Here's how the part is built. I have some questions about the finished solid (model axes, mm). Give positions to 0.01 mm unless a question says otherwise; leave off trailing zeros. Loops run counter-clockwise (first coordinate to the right, second up) from the corner with the lowest first, then second, coordinate; pieces in that order, holes last. Notation, with made-up numbers: (24, -40) -> (34, -40) arc R9 cw to (34, -32) -> close; hole circle Ø3 at (47, 32). An arc over 180 degrees is marked (long way). Answer in a Markdown table with one row per item. Add a question column.
Item 1: If I drill on line 1 (Y direction, x = 0, z = 0.3); line 2 (X direction, y = -1, z = 0.3); line 3 (X direction, y = 2, z = 0.9), over which ranges is the centre line in solid material (lowest first)?
Item 2: We'd pull the mould along X, two halves only. Please class faces 1 (the face through (0, -4, 1.05)), 2 (the face through (4.74, -2.79, 0.01)), 3 (the face through (-4.785, -2.712, 0.014)), 4 (the face through (0.45, 3.425, -0.015)): released by +X, released by -X, zero draft, split by the parting line, or undercut.
Item 3: If we section it at B-B (z = -0.05): Write out the boundary of the cut face in (x, y), then the cut area to 3 significant figures.
Item 4: If we section it at A-A (x = 0): Write out the boundary of the cut face in (y, z), then the cut area to 3 significant figures.
```python
from build123d import *

# Parameters (mm, degrees)
BOSS_EXTRUDE1_DEPTH      = 1.05
F_5_16_24_TAPPED_HOLE1_D = 6.9088


with BuildPart() as part:
    # Sketch2 → Boss-Extrude1 (new body, symmetric)
    with BuildSketch(Plane.XY):
        Polygon((-3.175426481, -5.5), (3.175426481, -5.5), (6.350852961, 0), (3.175426481, 5.5), (-3.175426481, 5.5), (-6.350852961, 0), align=None)
    extrude(amount=BOSS_EXTRUDE1_DEPTH, both=True)

    # 5/16-24 Tapped Hole1 (through all)
    with Locations(Plane.XY.offset(1.05)):
        with Locations((0, 0)):
            Hole(F_5_16_24_TAPPED_HOLE1_D / 2)

    # Sketch7 → Cut-Revolve2 (revolve, cut)
    with BuildSketch(Plane(origin=(0, 0, 0), x_dir=(1, 0, 0), z_dir=(0, 1, 0))):
        with BuildLine():
            Line((-6.350852961, -0.55), (-6.350852961, -1.05))
            Line((-6.350852961, -1.05), (-5.4, -1.05))
            ThreePointArc((-5.4, -1.05), (-5.921724154, -0.888044561), (-6.350852961, -0.55))
        make_face()
    cut_revolve2 = revolve(axis=Axis((0, 0, 0), (0, 0, 1)), mode=Mode.SUBTRACT)

    # Mirror1: Cut-Revolve2 across plane
    add(cut_revolve2.mirror(Plane.XY), mode=Mode.SUBTRACT)


solid = part.part
```
Recorded:
| question | item | result |
|---|---|---|
| 1 | line 1 | y = -5.5 to -3.45, 3.45 to 5.5 |
| 1 | line 2 | x = -5.77 to -3.31, 3.31 to 5.77 |
| 1 | line 3 | x = -5.2 to -2.82, 2.82 to 5.2 |
| 2 | face 1 | zero draft |
| 2 | face 2 | released by +X |
| 2 | face 3 | released by -X |
| 2 | face 4 | undercut |
| 3 | outline | (-6.35, 0) -> (-3.18, -5.5) -> (3.18, -5.5) -> (6.35, 0) -> (3.18, 5.5) -> (-3.18, 5.5) -> close; hole circle Ø6.91 at (0, 0) |
| 3 | area | 67.3 mm^2 |
| 4 | outline | (-5.5, -1.03) arc R1.5 ccw to (-5.4, -1.05) -> (-3.45, -1.05) -> (-3.45, 1.05) -> (-5.4, 1.05) arc R1.5 ccw to (-5.5, 1.03) -> close; (3.45, -1.05) -> (5.4, -1.05) arc R1.5 ccw to (5.5, -1.03) -> (5.5, 1.03) arc R1.5 ccw to (5.4, 1.05) -> (3.45, 1.05) -> close |
| 4 | area | 8.59 mm^2 |
